Model file for the job. Use its own axes, mm. A direction names the side the tool comes from. Round coordinates to 2 decimals unless told otherwise and drop trailing zeros. Loops run counter-clockwise (first coordinate to the right, second up) from the corner with the lowest first, then second, coordinate; pieces in that order, holes last. Notation, with made-up numbers: M 18,-29.5 L 40,-29.5 A21 ccw 40,-1.5 Z; hole C 80,-33.75 d1. An arc over 180 degrees is marked long. Use a Markdown table: item, result. Add a question column.
Q1. Cut at A-A (x = 309.88). Give the cut face in (y, z).
Q2. Cut at D-D (z = 2.54). State how many separate pieces and enclosed holes the cut face has, plus the area to 3 significant figures.
Q3. Cut at B-B (y = 10.16). Give the cut face in (x, z).
Q4. Cut at C-C (y = 86). Give the cut face in (x, z).
Q5. Pin check, flat tips, straight feed: pin 1 (5 mm diameter, centred on x = 84.35, y = 77.83, fed in from -Z); pin 2 (10 mm diameter, centred on x = 309.88, y = 107.95, fed in from +Z); pin 3 (1.7 mm diameter, centred on y = 156.21, z = 2.54, fed in from +X). Stop position of each tip, or through.
Q6. Tool access for faces 1 (the face through (250, 28, 1.27)), 2 (the face through (184, 141, 0)), 3 (the face through (238.89, 26.15, 2.5)): list every direction of +Z, -Z, +X, -X, +Y, -Y with a clear straight run to the whole face (end or side of a thin tool).
Q7. Mould opens along Y. For faces 4 (the face through (64.88, 101.75, 2.5)), 5 (the face through (86.08, 64.33, 2.5)), 6 (the face through (304.014, 105.518, 2.504)), 7 (the face through (243, 27, 0)) say: +Y half, -Y half, draft (parallel to the pull), parting line (faces both ways), or undercut.
Q8. Probe line 1 (X direction, y = 218.44, z = 1.05); line 2 (Y direction, x = 366.75, z = 2.54); line 3 (X direction, y = 119, z = 2.1). List the from-to ranges inside material, lowest first. Write a range as from..to.
from build123d import *

# Parameters (mm, degrees)
BOSS_EXTRUDE1_DEPTH = 5.08
CUT_EXTRUDE2_DEPTH  = 1.27
SKETCH5_W           = 38.1
SKETCH5_H           = 63.5
CUT_EXTRUDE3_DEPTH  = 7.62
SKETCH6_R           = 1.905
CUT_EXTRUDE4_DEPTH  = 7.62
SKETCH7_R           = 38.1
CUT_EXTRUDE5_DEPTH  = 7.62
SKETCH8_R           = 1.905
SKETCH8_W           = 88.9
SKETCH8_H           = 19.05
CUT_EXTRUDE6_DEPTH  = 7.62
SKETCH9_R           = 6.35
CUT_EXTRUDE7_DEPTH  = 7.62
SKETCH10_R          = 6.35
CUT_EXTRUDE8_DEPTH  = 7.62
SKETCH11_R          = 1.5
CUT_EXTRUDE9_DEPTH  = 25.4
SKETCH12_R          = 2
CUT_EXTRUDE10_DEPTH = 381
SKETCH13_R          = 1.4224
CUT_EXTRUDE11_DEPTH = 12.7


with BuildPart() as part:
    # Sketch2 → Boss-Extrude1 (new body)
    with BuildSketch(Plane.XY):
        Polygon((0, 0), (32.101676515, 0), (141.594783791, 130.488803961), (263.277562057, 0), (373.38, 0), (373.38, 228.6), (0, 228.6), align=None)
    extrude(amount=BOSS_EXTRUDE1_DEPTH)

    # Sketch4 → Cut-Extrude2 (cut)
    with BuildSketch(Plane(origin=(0, 0, 0), x_dir=(-1, 0, 0), z_dir=(0, 0, -1))):
        Polygon((-283.710082919, 0), (-271.867141325, 0), (-141.594783791, 139.7), (-24.372565316, 0), (-13.716, 0), (-141.594783791, 152.4), align=None)
    extrude(amount=-CUT_EXTRUDE2_DEPTH, mode=Mode.SUBTRACT)

    # Sketch5 → Cut-Extrude3 (cut)
    with BuildSketch(Plane.XY.offset(5.08)):
        with Locations((19.05, 95.25)):
            Rectangle(SKETCH5_W, SKETCH5_H)
    extrude(amount=-CUT_EXTRUDE3_DEPTH, mode=Mode.SUBTRACT)

    # Sketch6 → Cut-Extrude4 (cut)
    with BuildSketch(Plane(origin=(0, 0, 1.27), x_dir=(-1, 0, 0), z_dir=(0, 0, -1))):
        with Locations((-51.69789323, 38.91505771)):
            Circle(SKETCH6_R)
        with Locations((-84.351503802, 77.830115421)):
            Circle(SKETCH6_R)
        with Locations((-117.005114374, 116.745173131)):
            Circle(SKETCH6_R)
        with Locations((-167.57892131, 118.185423968)):
            Circle(SKETCH6_R)
        with Locations((-242.932920113, 37.378153476)):
            Circle(SKETCH6_R)
        with Locations((-260.255678459, 18.801769455)):
            Circle(SKETCH6_R)
    extrude(amount=-CUT_EXTRUDE4_DEPTH, mode=Mode.SUBTRACT)

    # Sketch7 → Cut-Extrude5 (cut)
    with BuildSketch(Plane(origin=(0, 0, 0), x_dir=(-1, 0, 0), z_dir=(0, 0, -1))):
        with Locations((-202.206417984, 87.401980028)):
            Circle(SKETCH7_R)
    extrude(amount=-CUT_EXTRUDE5_DEPTH, mode=Mode.SUBTRACT)

    # Sketch8 → Cut-Extrude6 (cut)
    with BuildSketch(Plane(origin=(0, 0, 0), x_dir=(-1, 0, 0), z_dir=(0, 0, -1))):
        with Locations((-132.08, 212.598)):
            Circle(SKETCH8_R)
        with Locations((-30.48, 212.598)):
            Circle(SKETCH8_R)
        with Locations((-132.08, 161.798)):
            Circle(SKETCH8_R)
        with Locations((-30.48, 161.798)):
            Circle(SKETCH8_R)
        with Locations((-81.28, 203.073)):
            Rectangle(SKETCH8_W, SKETCH8_H)
    extrude(amount=-CUT_EXTRUDE6_DEPTH, mode=Mode.SUBTRACT)

    # Sketch9 → Cut-Extrude7 (cut)
    with BuildSketch(Plane(origin=(0, 0, 0), x_dir=(-1, 0, 0), z_dir=(0, 0, -1))):
        with Locations((-327.914, 10.16)):
            Circle(SKETCH9_R)
        with Locations((-280.139109994, 96.938127918)):
            Circle(SKETCH9_R)
        with Locations((-212.580352446, 169.3860256)):
            Circle(SKETCH9_R)
    extrude(amount=-CUT_EXTRUDE7_DEPTH, mode=Mode.SUBTRACT)

    # Sketch10 → Cut-Extrude8 (cut)
    with BuildSketch(Plane(origin=(0, 0, 0), x_dir=(-1, 0, 0), z_dir=(0, 0, -1))):
        with Locations((-309.88, 107.95)):
            Circle(SKETCH10_R)
        with Locations((-63.5, 107.95)):
            Circle(SKETCH10_R)
    extrude(amount=-CUT_EXTRUDE8_DEPTH, mode=Mode.SUBTRACT)

    # Sketch11 → Cut-Extrude9 (cut)
    with BuildSketch(Plane(origin=(0, 0, 0), x_dir=(-1, 0, 0), z_dir=(0, 0, -1))):
        with Locations((-345.44, 218.44)):
            Circle(SKETCH11_R)
        with Locations((-281.94, 218.44)):
            Circle(SKETCH11_R)
        with Locations((-218.44, 218.44)):
            Circle(SKETCH11_R)
        with Locations((-2.54, 218.44)):
            Circle(SKETCH11_R)
    extrude(amount=-CUT_EXTRUDE9_DEPTH, mode=Mode.SUBTRACT)

    # Sketch12 → Cut-Extrude10 (cut)
    with BuildSketch(Plane.XY.offset(5.08)):
        with Locations((322.58, 132.08)):
            Circle(SKETCH12_R)
        with Locations((271.78, 132.08)):
            Circle(SKETCH12_R)
        with Locations((220.98, 132.08)):
            Circle(SKETCH12_R)
        with Locations((119.38, 132.08)):
            Circle(SKETCH12_R)
        with Locations((68.58, 132.08)):
            Circle(SKETCH12_R)
    extrude(amount=-CUT_EXTRUDE10_DEPTH, mode=Mode.SUBTRACT)

    # Sketch13 → Cut-Extrude11 (cut)
    with BuildSketch(Plane(origin=(373.38, 0, 0), x_dir=(0, 0, -1), z_dir=(1, 0, 0))):
        with Locations((-2.54, 203.2)):
            Circle(SKETCH13_R)
        with Locations((-2.54, 156.21)):
            Circle(SKETCH13_R)
    extrude(amount=-CUT_EXTRUDE11_DEPTH, mode=Mode.SUBTRACT)


solid = part.part
Checked values:
| question | item | result |
|---|---|---|
| 1 | outline | M 0,0 L 101.6,0 L 101.6,5.08 L 0,5.08 Z; M 114.3,0 L 228.6,0 L 228.6,5.08 L 114.3,5.08 Z |
| 2 | separate pieces | 1 |
| 2 | enclosed holes | 25 |
| 2 | area | 61,900 mm^2 |
| 3 | outline | M 0,0 L 22.24,0 L 22.24,1.27 L 32.9,1.27 L 32.9,0 L 40.63,0 L 40.63,5.08 L 0,5.08 Z; M 253.8,0 L 262.39,0 L 262.39,1.27 L 274.24,1.27 L 274.24,0 L 321.56,0 L 321.56,5.08 L 253.8,5.08 Z; M 334.26,0 L 373.38,0 L 373.38,5.08 L 334.26,5.08 Z |
| 4 | outline | M 38.1,0 L 85.88,0 L 85.88,1.27 L 96.54,1.27 L 96.54,0 L 104.26,0 L 104.26,5.08 L 38.1,5.08 Z; M 240.28,0 L 373.38,0 L 373.38,5.08 L 240.28,5.08 Z |
| 5 | pin 1 | stops at z = 1.27 |
| 5 | pin 2 | passes through |
| 5 | pin 3 | stops at x = 360.68 |
| 6 | face 1 | -Z |
| 6 | face 2 | -Z, +X, -X, +Y, -Y |
| 6 | face 3 | +Z, -Z, -Y |
| 7 | face 4 | undercut |
| 7 | face 5 | -Y half |
| 7 | face 6 | undercut |
| 7 | face 7 | draft |
| 8 | line 1 | x = 0..1.04, 4.04..216.94, 219.94..280.44, 283.44..343.94, 346.94..373.38 |
| 8 | line 2 | y = 0..154.79, 157.63..201.78, 204.62..228.6 |
| 8 | line 3 | x = 38.1..131.95, 152.31..165.86, 169.3..180.92, 223.49..373.38 |
